Design review of the part shown in the three views and the two pictorial views. Dimensions are in mm from the part's minimum x, y and z. A direction names the side the tool comes from. Round coordinates to 2 decimals unless told otherwise and drop trailing zeros. Order: outer loops, then holes, each group sorted by start corner. A loop starts at its lowest first (then second) coordinate and runs counter-clockwise, first axis right, second up.
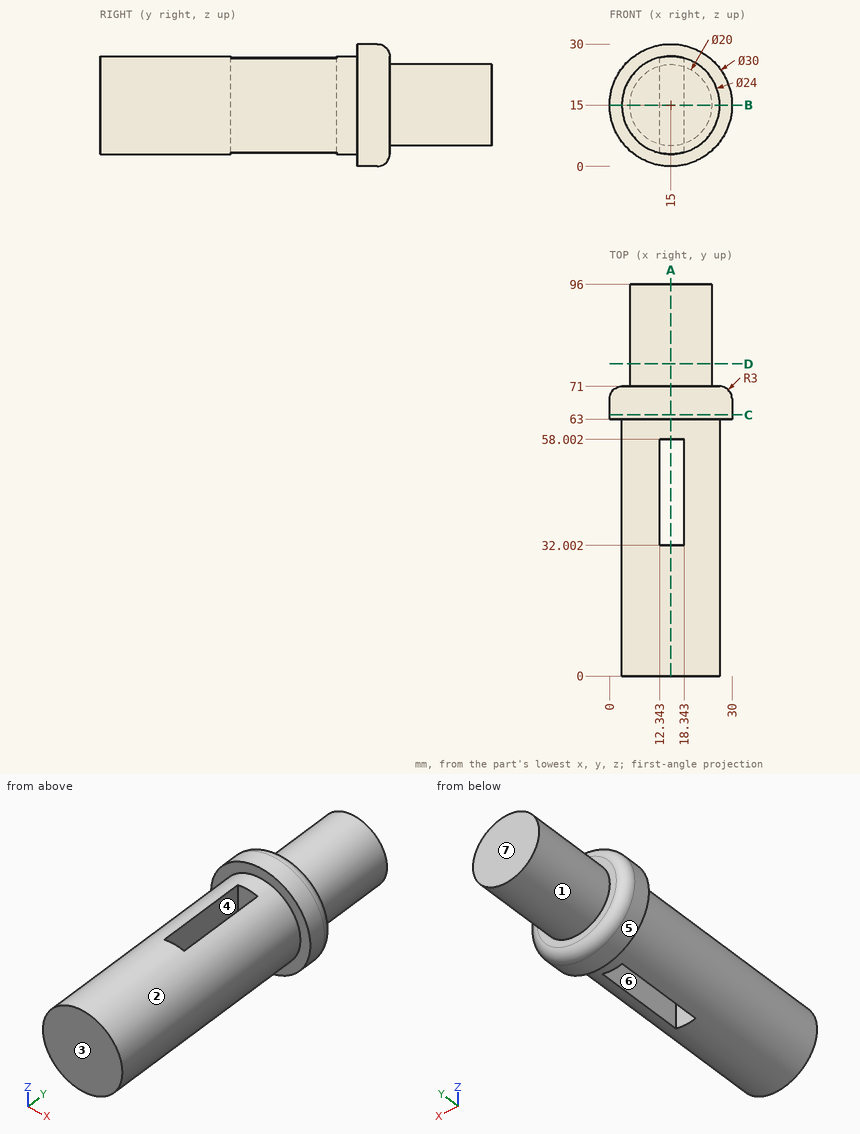
(1) Add section B-B on z = 15. Give the boundary of the cut face in (x, y).
(2) Draft analysis for pull direction Y (two halves, no side actions). For the marked faces 4, 5, 6 and 7, state which applies: pulls with the +Y half, pulls with the -Y half, needs draft (parallel to the pull), parting line crosses it, or undercut.
(3) Tool access review of the marked faces 1, 2 and 3: name each direction out of +Z, -Z, +X, -X, +Y, -Y from which nothing blocks a thin tool from reaching the whole face with its end or side.
(4) Add section D-D on y = 76.5. Give the boundary of the cut face in (x, z), plus the area to 3 significant figures.
(5) Add section A-A on x = 15. Give the boundary of the cut face in (y, z), plus the area to 3 significant figures.
(6) Wall thickness on L1, parallel to X at y = 33, z = 14.5; L2, parallel to Y at x = 13.5, z = 24; L3, parallel to Y at x = 23.75, z = 6.75: over which ranges is each line inside the solid? List them lowest first.
(7) Clearance check with flat-ended pins moving along their axes: P1, Ø5, axis at y = 42.5, z = 8, coming from the -X side; P2, Ø3, axis at x = 3, z = 23.5, coming from the +Y side; P3, Ø8, axis at x = 8.5, z = 16, coming from the -Y side; P4, Ø11.5, axis at y = 46.5, z = 11, coming from the -X side. State where each tip first meets the part, or that it passes through.
(8) Add section C-C on y = 64. Give the boundary of the cut face in (x, z), plus the area to 3 significant figures.
Here are the results:
1. outline: (0, 63) - (3, 63) - (3, 0) - (27, 0) - (27, 63) - (30, 63) - (30, 68) arc R3 ccw to (27, 71) - (25, 71) - (25, 96) - (5, 96) - (5, 71) - (3, 71) arc R3 ccw to (0, 68) - close; hole (12.34, 32) - (18.34, 32) - (18.34, 58) - (12.34, 58) - close
2. face 4: undercut
2. face 5: needs draft
2. face 6: undercut
2. face 7: pulls with the +Y half
3. face 1: +Y
3. face 2: -Y
3. face 3: +Z, -Z, +X, -X, -Y
4. outline: circle Ø20 at (15, 15)
4. area: 314 mm2
5. outline: (0, 3) - (32, 3) - (32, 27) - (0, 27) - close; (58, 3) - (63, 3) - (63, 0) - (68, 0) arc R3 ccw to (71, 3) - (71, 5) - (96, 5) - (96, 25) - (71, 25) - (71, 27) arc R3 ccw to (68, 30) - (63, 30) - (63, 27) - (58, 27) - close
5. area: 1,620 mm2
6. L1: x = 3.01 to 12.34, 18.34 to 26.99
6. L2: y = 0 to 32, 58 to 96
6. L3: y = 63 to 71
7. P1: stops at x = 3.88
7. P2: stops at y = 70.75
7. P3: stops at y = 0
7. P4: stops at x = 3
8. outline: circle Ø30 at (15, 15)
8. area: 707 mm2
